Input: part model. Units: mm. Frame: model coordinates. A direction names the side the tool comes from. Give positions to 0.01 mm unless a question says otherwise; leave off trailing zeros. Loops run counter-clockwise (first coordinate to the right, second up) from the corner with the lowest first, then second, coordinate; pieces in that order, holes last. Notation, with made-up numbers: (61, 22) -> (108, 22) arc R15 ccw to (108, 43) -> close; hole circle Ø8 at (-4.5, 77). An arc over 180 degrees is marked (long way). Answer as a JSON object with one key per item and string values.
```python
from build123d import *

# Parameters (mm, degrees)
BOSS_EXTRUDE1_DEPTH              = 3.175
M2_5_CLEARANCE_HOLE1_D           = 2.7
M2_5_CLEARANCE_HOLE1_CSINK_D     = 2.75
M2_5_CLEARANCE_HOLE1_CSINK_ANGLE = 100
FILLET1_R                        = 0.25


with BuildPart() as part:
    # Sketch1 → Boss-Extrude1 (new body)
    with BuildSketch(Plane.XY):
        with BuildLine():
            Line((-12.5, 4), (-12.5, 0))
            ThreePointArc((-12.5, 0), (0, -12.5), (12.5, 0))
            Line((12.5, 0), (12.5, 4))
            Line((12.5, 4), (1.8375, 4))
            Line((1.8375, 4), (1.8375, -0.5))
            Line((1.8375, -0.5), (-1.8375, -0.5))
            Line((-1.8375, -0.5), (-1.8375, 4))
            Line((-1.8375, 4), (-12.5, 4))
        make_face()
    extrude(amount=BOSS_EXTRUDE1_DEPTH)

    # M2.5 Clearance Hole1 (through all)
    with Locations(Plane.XY.offset(3.175)):
        with Locations((-7.5, 0), (7.5, 0)):
            CounterSinkHole(M2_5_CLEARANCE_HOLE1_D / 2, M2_5_CLEARANCE_HOLE1_CSINK_D / 2, counter_sink_angle=M2_5_CLEARANCE_HOLE1_CSINK_ANGLE)

    # Fillet1
    fillet1_edges = [part.edges().sort_by_distance(p)[0] for p in [
        (-12.5, 4, 1.5875),
        (-1.8375, 4, 1.5875),
        (-1.8375, -0.5, 1.5875),
        (1.8375, -0.5, 1.5875),
        (1.8375, 4, 1.5875),
        (12.5, 4, 1.5875),
    ]]
    fillet(fillet1_edges, radius=FILLET1_R)


solid = part.part
```
Q1. Section B-B, the plane x = 7.5. Return the cut outline in (y, z) (3 decimals), then the cut area to 3 significant figures.
Evaluation:
{"outline": "(-10, 0) -> (-1.35, 0) -> (-1.35, 3.154) -> (-1.375, 3.175) -> (-10, 3.175) -> close; (1.35, 0) -> (4, 0) -> (4, 3.175) -> (1.375, 3.175) -> (1.35, 3.154) -> close", "area": "35.9 mm2"}
Q2. Section A-A, the plane z = 2.3. Return the cut outline in (x, y), then the cut area to 3 significant figures.
Evaluation:
{"outline": "(-12.5, 0) arc R12.5 ccw to (12.5, 0) -> (12.5, 3.75) arc R0.25 ccw to (12.25, 4) -> (2.09, 4) arc R0.25 ccw to (1.84, 3.75) -> (1.84, -0.25) arc R0.25 cw to (1.59, -0.5) -> (-1.59, -0.5) arc R0.25 cw to (-1.84, -0.25) -> (-1.84, 3.75) arc R0.25 ccw to (-2.09, 4) -> (-12.25, 4) arc R0.25 ccw to (-12.5, 3.75) -> close; hole circle Ø2.7 at (-7.5, 0); hole circle Ø2.7 at (7.5, 0)", "area": "317 mm2"}
Q3. Section D-D, the plane y = -8.25. Return the cut outline in (x, z) (3 decimals).
Evaluation:
{"outline": "(-9.391, 0) -> (9.391, 0) -> (9.391, 3.175) -> (-9.391, 3.175) -> close"}
Q4. Ray query, line 1 along X through (y, z) = (0, 2.3); line 2 along X through (y, z) = (3, 0.8); line 3 along X through (y, z) = (-1, 0.2). Return the intervals inside material, ascending.
Evaluation:
{"line 1": "x = -12.5 to -8.85, -6.15 to -1.84, 1.84 to 6.15, 8.85 to 12.5", "line 2": "x = -12.5 to -1.84, 1.84 to 12.5", "line 3": "x = -12.46 to -8.41, -6.59 to 6.59, 8.41 to 12.46"}
Q5. Access query for faces 1 (the flat face through (-1.838, 2, 2)), 2 (the flat face through (7, 4, 2)). Directions: +Z, -Z, +X, -X, +Y, -Y. A direction counts if a zero-diameter tool reaches every point of the face in a straight line with its end or side. Return the directions, or none.
Evaluation:
{"face 1": "+Z, -Z, +Y", "face 2": "+Z, -Z, +X, -X, +Y"}
Q6. Section C-C, the plane x = 0. Return the cut outline in (y, z) (3 decimals), then the cut area to 3 significant figures.
Evaluation:
{"outline": "(-12.5, 0) -> (-0.5, 0) -> (-0.5, 3.175) -> (-12.5, 3.175) -> close", "area": "38.1 mm2"}
Q7. Pin query (flat end, axial travel): pin 1 (1.5 mm diameter, centred on y = -3.5, z = 2.5, fed in from +X). Return the tip coordinate at first contact, or that it passes through.
Evaluation:
{"pin 1": "stops at x = 12.19"}
